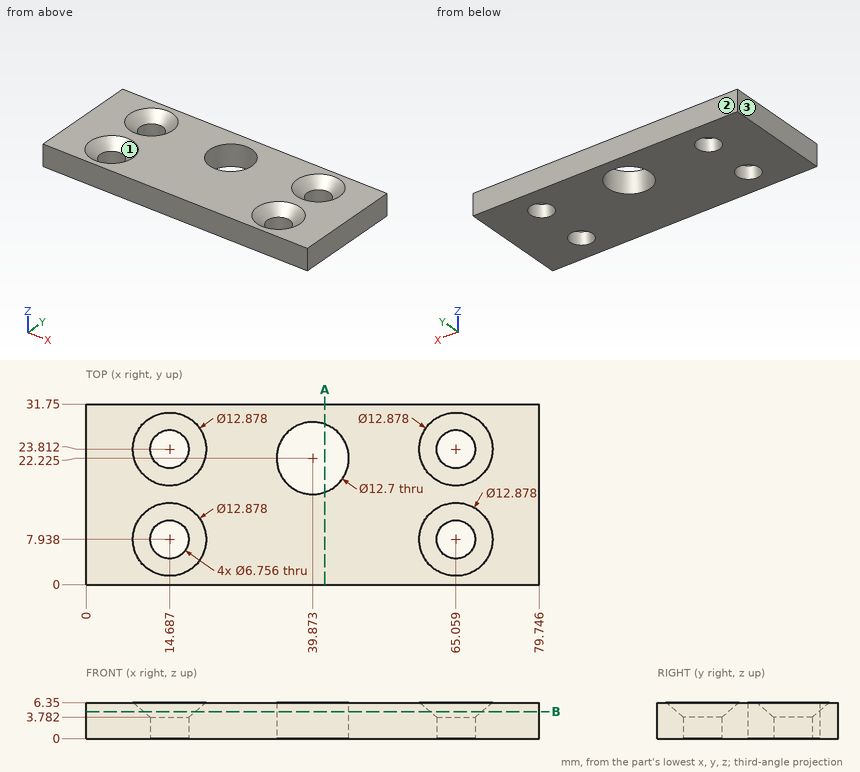
Check sheet for the drawn part. Datum: minimum x, y, z corner. Units: mm. Give positions to 0.01 mm unless a question says otherwise; leave off trailing zeros. Order: outer loops, then holes, each group sorted by start corner. A loop starts at its lowest first (then second) coordinate and runs counter-clockwise, first axis right, second up. Notation, with made-up numbers: (26, 69.25) - (61, 69.25) arc R20 cw to (61, 98.25) - close; hole circle Ø8 at (-17.5, 47.25). An arc over 180 degrees is marked (long way). Answer in a Markdown table with one row per item. Add a question column.
Q1. Cross-section at A-A, the plane x = 42. Enter the section's corners in (y, z).
Q2. Cross-section at B-B, the plane z = 4.75. Count the separate pieces of the cut face and the enclosed holes in it, then the cut area to 3 significant figures.
Q3. Gauge pin test, flat end, axial feed: pin 1 (11 mm diameter, centred on x = 14.69, y = 23.81, fed in from +Z) (1 decimal). Record the tip position at first contact, or that the pin passes through.
Q4. Material ranges on probe 1 along X at (y, z) = (9.5, 2.5) (1 decimal); probe 2 along X at (y, z) = (25.5, 5.75) (1 decimal); probe 3 along X at (y, z) = (22, 3.5) (1 decimal), recorded low to high. Write a range as from..to.
Q5. Mould release check, pull along X, two halves, no side actions. Record for the marked faces 1, 2 and 3: pulls with the +X half, pulls with the -X half, needs draft (parallel to the pull), parting line crosses it, or undercut.
Check values:
| question | item | result |
|---|---|---|
| 1 | outline | (0, 0) - (16.24, 0) - (16.24, 6.35) - (0, 6.35) - close; (28.21, 0) - (31.75, 0) - (31.75, 6.35) - (28.21, 6.35) - close |
| 2 | separate pieces | 1 |
| 2 | enclosed holes | 5 |
| 2 | area | 2,150 mm^2 |
| 3 | pin 1 | stops at z = 5.6 |
| 4 | probe 1 | x = 0..11.7, 17.7..62.1, 68.1..79.7 |
| 4 | probe 2 | x = 0..9.2, 20.2..34.4, 45.3..59.6, 70.5..79.7 |
| 4 | probe 3 | x = 0..11.8, 17.5..33.5, 46.2..62.2, 67.9..79.7 |
| 5 | face 1 | undercut |
| 5 | face 2 | needs draft |
| 5 | face 3 | pulls with the -X half |
